Verification items for the finished model (mm, model axes). A direction names the side the tool comes from. Coordinates: 2 decimals unless noted, no trailing zeros. Write each loop counter-clockwise with the first axis right and the second up, starting at its lowest first coordinate (ties: lowest second). Pieces come first, ordered by that corner, then holes. Notation, with made-up numbers: M 52,10 L 73,10 A14 cw 73,33 Z; hole C -22.75,37.5 d7. An arc over 180 degrees is marked long. One line per item, written item: value.
```python
from build123d import *

# Parameters (mm, degrees)
F0_R      = 76.2
F1_DEPTH  = 25.4
F4_R      = 19.05
F5_DEPTH  = 12.7
F7_R      = 19.05
F8_DEPTH  = 12.7
F9_R      = 19.05
F10_DEPTH = 12.7
F11_R     = 19.05
F12_DEPTH = 12.7


with BuildPart() as f1:
    # F0 (on Top) → F1 (new body)
    with BuildSketch(Plane.XY):
        Circle(F0_R)
    extrude(amount=F1_DEPTH)

    # F4 (on plane+point) → F5 (join, symmetric)
    with BuildSketch(Plane.XZ.offset(-31.75)):
        with Locations((38.4162291884, 25.6418008357)):
            Circle(F4_R)
    extrude(amount=F5_DEPTH, both=True)

    # F7 (on plane+point) → F8 (join, symmetric)
    with BuildSketch(Plane.XZ.offset(31.75)):
        with Locations((37.968441844, 25.2595245838)):
            Circle(F7_R)
    extrude(amount=F8_DEPTH, both=True)

    # F9 (on plane+point) → F10 (join, symmetric)
    with BuildSketch(Plane.XZ.offset(-31.75)):
        with Locations((-38.3299067616, 25.1507181674)):
            Circle(F9_R)
    extrude(amount=F10_DEPTH, both=True)

    # F11 (on plane+point) → F12 (join, symmetric)
    with BuildSketch(Plane.XZ.offset(31.75)):
        with Locations((-39.1971170902, 27.3897647858)):
            Circle(F11_R)
    extrude(amount=F12_DEPTH, both=True)


solid = f1.part
```
Item 1: Cross-section at C-C, the plane y = 0. Enter the section's corners in (x, z).
The answers:
outline: M -76.2,0 L 76.2,0 L 76.2,25.4 L -76.2,25.4 Z
Item 2: Cross-section at D-D, the plane z = 17. Enter the section's corners in (x, y).
The answers:
outline: C 0,0 d152.4
Item 3: Access from +Z, -Z, +X, -X, +Y, -Y to the whole of each face (thin tool, end or side, straight path). Record for faces 4 (the face through (-1, 1, 0)), 5 (the face through (-39, 19.05, 33)), 6 (the face through (-39, -44.45, 34)), 7 (the face through (-39, 44.45, 33)), 8 (the face through (-37.914, 31.572, 44.196)).
The answers:
face 4: -Z, +X, -X, +Y, -Y
face 5: +Z, +X, -X
face 6: +Z, +X, -X, -Y
face 7: +Z, +X, -X, +Y
face 8: +Z, +Y
Item 4: Draft check along X on faces 1 (the face through (38.385, -31.928, 44.305)), 2 (the face through (-60.47, -46.367, 12.522)), 3 (the face through (38, -19.05, 33)). Enter one of: released by +X, released by -X, zero draft, split by the parting line, or undercut.
The answers:
face 1: undercut
face 2: split by the parting line
face 3: zero draft
Item 5: Cross-section at B-B, the plane x = 25. Enter the section's corners in (y, z), and give its area (3 significant figures).
The answers:
outline: M -71.98,0 L 71.98,0 L 71.98,25.4 L 44.45,25.4 L 44.45,39.17 L 19.05,39.17 L 19.05,25.4 L -19.05,25.4 L -19.05,39.21 L -44.45,39.21 L -44.45,25.4 L -71.98,25.4 Z
area: 4,360 mm²
Item 6: Cross-section at A-A, the plane z = 36.5. Enter the section's corners in (x, y).
The answers:
outline: M -55.93,-44.45 L -22.47,-44.45 L -22.47,-19.05 L -55.93,-19.05 Z; M -53.63,19.05 L -23.03,19.05 L -23.03,44.45 L -53.63,44.45 Z; M 22.59,-44.45 L 53.35,-44.45 L 53.35,-19.05 L 22.59,-19.05 Z; M 22.76,19.05 L 54.07,19.05 L 54.07,44.45 L 22.76,44.45 Z
Item 7: Scan lines: line 1 (Y direction, x = -36.5, z = 29.5); line 2 (Z direction, x = 15.5, y = 26.5); line 3 (X direction, y = -0.5, z = 8.5). Record each from-to range of solid material in increasing order.
The answers:
line 1: y = -44.45 to -19.05, 19.05 to 44.45
line 2: z = 0 to 25.4
line 3: x = -76.2 to 76.2
Item 8: Go/stop test with flat-tipped pins: P1, Ø5.5, axis at x = 37.5, z = 33.5, coming from the -Y side; P2, Ø23, axis at x = -30, z = 31, coming from the -Y side; P3, Ø5, axis at x = 13.5, z = 30, coming from the +Y side; P4, Ø12, axis at x = 35, z = 7.5, coming from the -Y side. Record where each tip stops, or that it passes through.
The answers:
P1: stops at y = -44.45
P2: stops at y = -73.54
P3: passes through
P4: stops at y = -70.47
